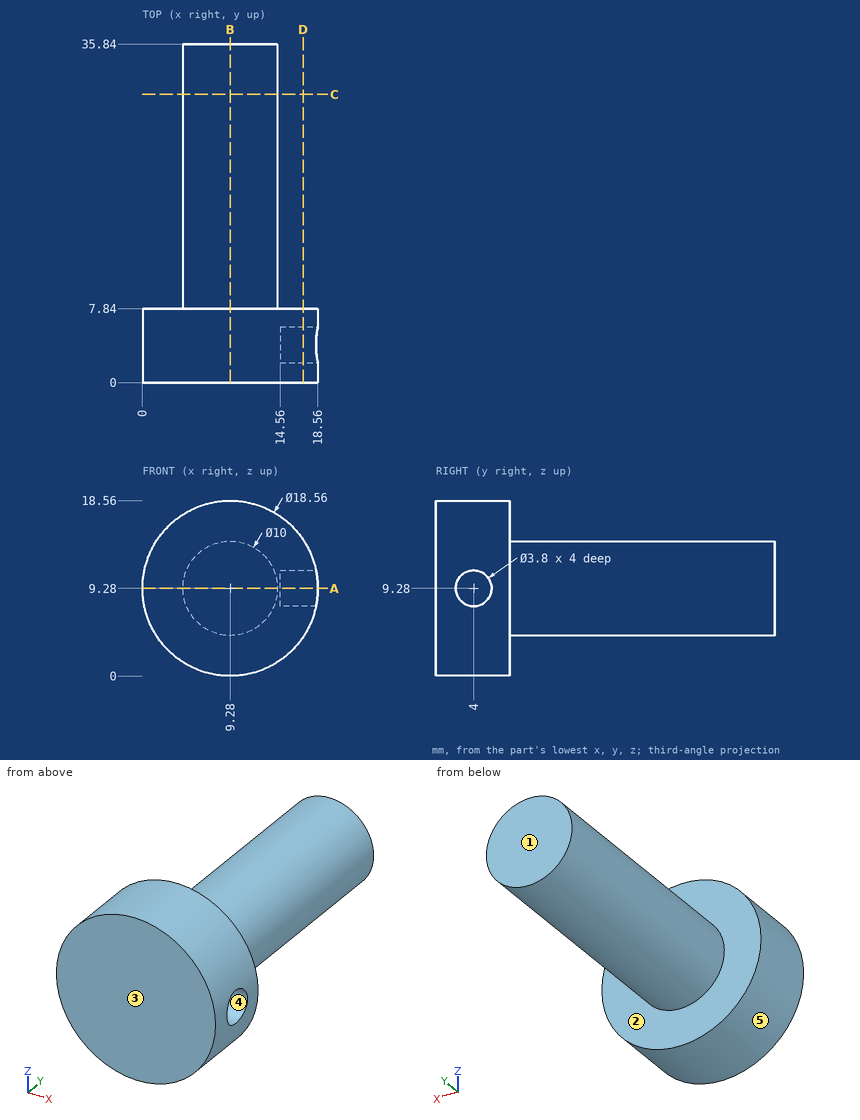
Input: dimensioned drawing with shaded views. Units: mm. Origin: part minimum x, y, z. A direction names the side the tool comes from. Give positions to 0.01 mm unless a question says otherwise; leave off trailing zeros. Order: outer loops, then holes, each group sorted by start corner. A loop starts at its lowest first (then second) coordinate and runs counter-clockwise, first axis right, second up. Notation, with made-up numbers: (28.5, 49) -> (45.5, 49) arc R25 ccw to (45.5, 65) -> close; hole circle Ø3 at (-2.5, 70). An arc over 180 degrees is marked (long way). Use a Markdown table: item, result.
1) Section query C-C, the plane y = 30.5. Return the cut outline in (x, z).
Answer list:
| item | result |
|---|---|
| outline | circle Ø10 at (9.28, 9.28) |
2) Section query B-B, the plane x = 9.28. Return the cut outline in (y, z).
Answer list:
| item | result |
|---|---|
| outline | (0, 0) -> (7.84, 0) -> (7.84, 4.28) -> (35.84, 4.28) -> (35.84, 14.28) -> (7.84, 14.28) -> (7.84, 18.56) -> (0, 18.56) -> close |
3) Section query A-A, the plane z = 9.28. Return the cut outline in (x, y), then the cut area to 3 significant figures.
Answer list:
| item | result |
|---|---|
| outline | (0, 0) -> (18.56, 0) -> (18.56, 2.1) -> (14.56, 2.1) -> (14.56, 5.9) -> (18.56, 5.9) -> (18.56, 7.84) -> (14.28, 7.84) -> (14.28, 35.84) -> (4.28, 35.84) -> (4.28, 7.84) -> (0, 7.84) -> close |
| area | 410 mm² |
4) Ray query, line 1 along Y through (x, z) = (16.7, 9.28); line 2 along Y through (x, z) = (6.75, 2.75); line 3 along X through (y, z) = (13, 9.5). Return the intervals inside material, ascending. Write a range as [from, to].
Answer list:
| item | result |
|---|---|
| line 1 | [0, 2.1], [5.9, 7.84] |
| line 2 | [0, 7.84] |
| line 3 | [4.28, 14.28] |
5) Reachability of the marked faces 1 and 2 from +Z, -Z, +X, -X, +Y, -Y: full face, straight path, thin tool, end or side. Return the list, or none.
Answer list:
| item | result |
|---|---|
| face 1 | +Z, -Z, +X, -X, +Y |
| face 2 | +Y |
6) Mould query, pull axis Z, two halves, no side actions, for the marked faces 3, 4 and 5. Classes: +Z half, -Z half, draft (parallel to the pull), parting line (faces both ways), or undercut.
Answer list:
| item | result |
|---|---|
| face 3 | draft |
| face 4 | undercut |
| face 5 | parting line |
7) Section query D-D, the plane x = 17. Return the cut outline in (y, z).
Answer list:
| item | result |
|---|---|
| outline | (0, 4.13) -> (7.84, 4.13) -> (7.84, 14.43) -> (0, 14.43) -> close; hole circle Ø3.8 at (4, 9.28) |
8) Contact query for flat-ended pins moving along their axis: P1, Ø1.9, axis at y = 3.5, z = 10, coming from the +X side; P2, Ø8, axis at y = 19, z = 15, coming from the -X side; P3, Ø1, axis at x = 8, y = 15, coming from the +Z side. Output: stop coordinate, or through.
Answer list:
| item | result |
|---|---|
| P1 | x = 14.56 |
| P2 | x = 4.59 |
| P3 | z = 14.22 |
